```python
from build123d import *

# Parameters (mm, degrees)
SKETCH1_W           = 127
SKETCH1_H           = 61.9252
BOSS_EXTRUDE1_DEPTH = 44.45
SKETCH1_3_W         = 127
SKETCH1_3_H         = 1.8415
CUT_EXTRUDE2_DEPTH  = 38.1
SKETCH2_W           = 71.12
SKETCH2_H           = 32.258
SKETCH2_W_2         = 35.442647017
SKETCH2_H_2         = 23.182829488
CUT_EXTRUDE3_DEPTH  = 38.1
CHAMFER2_SIZE       = 10.16
CUT_EXTRUDE5_DEPTH  = 100.210800294
FILLET3_R           = 2.54
SKETCH2_3_W         = 35.442647017
SKETCH2_3_H         = 23.182829488
CUT_EXTRUDE6_DEPTH  = 84.466970107
CHAMFER3_SIZE       = 2.54


with BuildPart() as part:
    # Sketch1 → Boss-Extrude1 (new body)
    with BuildSketch(Plane(origin=(0, 0, 0), x_dir=(1, 0, 0), z_dir=(0, 1, 0))):
        Rectangle(SKETCH1_W, SKETCH1_H)
    extrude(amount=BOSS_EXTRUDE1_DEPTH)

    # Sketch1<3> → Cut-Extrude2 (cut)
    with BuildSketch(Plane(origin=(0, 0, 0), x_dir=(1, 0, 0), z_dir=(0, 1, 0))):
        with Locations((0, 23.69185)):
            Rectangle(SKETCH1_3_W, SKETCH1_3_H)
        with Locations((0, -23.69185)):
            Rectangle(SKETCH1_3_W, SKETCH1_3_H)
    extrude(amount=CUT_EXTRUDE2_DEPTH, mode=Mode.SUBTRACT)

    # Sketch2 → Cut-Extrude3 (cut)
    with BuildSketch(Plane(origin=(0, 44.45, 0), x_dir=(1, 0, 0), z_dir=(0, 1, 0))):
        with Locations((1.016, 0)):
            Rectangle(SKETCH2_W, SKETCH2_H)
        with Locations((12.504676492, 0)):
            Rectangle(SKETCH2_W_2, SKETCH2_H_2, mode=Mode.SUBTRACT)
    extrude(amount=-CUT_EXTRUDE3_DEPTH, mode=Mode.SUBTRACT)

    # Chamfer2
    chamfer2_edges = [part.edges().sort_by_distance(p)[0] for p in [
        (36.576, 44.45, 0),
        (1.016, 44.45, -16.129),
        (-34.544, 44.45, 0),
        (1.016, 44.45, 16.129),
    ]]
    chamfer(chamfer2_edges, length=CHAMFER2_SIZE)

    # Sketch7 → Cut-Extrude5 (cut, through all)
    with BuildSketch(Plane.XY.offset(30.9626)):
        Polygon((-50.795476794, 0), (-63.5, 44.45), (-63.5, 0), align=None)
        Polygon((63.5, 44.45), (50.795476794, 0), (63.5, 0), align=None)
    extrude(amount=-CUT_EXTRUDE5_DEPTH, mode=Mode.SUBTRACT)

    # Fillet3
    fillet3_edges = [part.edges().sort_by_distance(p)[0] for p in [
        (-57.147738397, 22.225, -30.9626),
        (-57.147738397, 22.225, 30.9626),
        (57.147738397, 22.225, 30.9626),
        (57.147738397, 22.225, -30.9626),
    ]]
    fillet(fillet3_edges, radius=FILLET3_R)

    # Sketch2<3> → Cut-Extrude6 (cut, through all)
    with BuildSketch(Plane(origin=(0, 44.45, 0), x_dir=(1, 0, 0), z_dir=(0, 1, 0))):
        with Locations((12.504676492, 0)):
            Rectangle(SKETCH2_3_W, SKETCH2_3_H)
    extrude(amount=-CUT_EXTRUDE6_DEPTH, mode=Mode.SUBTRACT)

    # Chamfer3
    chamfer3_edges = [part.edges().sort_by_distance(p)[0] for p in [
        (30.226, 0, 0),
        (12.504676491, 0, 11.591414744),
        (-5.216647017, 0, 0),
        (12.504676491, 0, -11.591414744),
    ]]
    chamfer(chamfer3_edges, length=CHAMFER3_SIZE)


solid = part.part
```
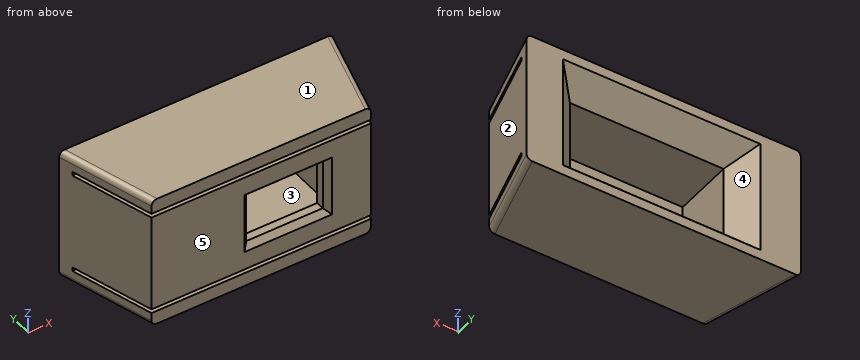
Build history of the part. All positions in model axes, mm. Face numbers are marked on the shaded views. A direction names the side the tool comes from. Round coordinates to 2 decimals unless told otherwise and drop trailing zeros. Write each loop counter-clockwise with the first axis right and the second up, starting at its lowest first coordinate (ties: lowest second). Pieces come first, ordered by that corner, then holes.
1) Band-saw the part on C-C, the plane y = 17. Give the number of separate pieces and of enclosed holes in the cut face, and give its area (3 significant figures).
2) Band-saw the part on A-A, the plane x = 23.5. List the corners of the cut face in (y, z).
3) Band-saw the part on D-D, the plane z = 20. List the corners of the cut face in (x, y) (3 decimals), and give its area (3 significant figures).
4) 3-axis set-ups, long thin cutter, end or side, ignore diameter. For the marked faces 4 and 5: which of +Z, -Z, +X, -X, +Y, -Y reach the whole face in a straight line?
5) Pin check, flat tips, straight feed: pin 1 (14 mm diameter, centred on y = 22, z = -1, fed in from -X); pin 2 (0.6 mm diameter, centred on x = 18.5, z = -23.5, fed in from -Y); pin 3 (3 mm diameter, centred on y = 4.5, z = -1, fed in from -X). Stop position of each tip, or through.
6) Band-saw the part on B-B, the plane x = -46. List the corners of the cut face in (y, z).
7) Drill centre lines: probe 1 along Z at (x, y) = (57, 37.5); probe 2 along Z at (x, y) = (-18, 15); probe 3 along Z at (x, y) = (-2, 6). Where is each one in solid material? Low to high.
8) Mould opens along X. For the marked faces 1, 2 and 3 say: +X half, -X half, draft (parallel to the pull), parting line (faces both ways), or undercut.
Ans:
1. separate pieces: 3
1. enclosed holes: 1
1. area: 4,180 mm2
2. outline: (0, -30.96) - (44.45, -30.96) - (44.45, -26.29) - (34.29, -16.13) - (6.35, -16.13) - (6.35, -11.59) - (2.54, -11.59) - (0, -14.13) - (0, -22.77) - (38.1, -22.77) - (38.1, -24.61) - (0, -24.61) - close; (0, 14.13) - (2.54, 11.59) - (6.35, 11.59) - (6.35, 16.13) - (34.29, 16.13) - (44.45, 26.29) - (44.45, 30.96) - (0, 30.96) - (0, 24.61) - (38.1, 24.61) - (38.1, 22.77) - (0, 22.77) - close
3. outline: (-63.5, 44.45) - (-50.795, 0) - (50.795, 0) - (63.5, 44.45) - (46.736, 44.45) - (40.447, 38.161) - (-38.415, 38.161) - (-44.704, 44.45) - close
3. area: 4,540 mm2
4. face 4: +Y
4. face 5: +Z, -Z, +X, -X, -Y
5. pin 1: stops at x = -59.08
5. pin 2: stops at y = 38.1
5. pin 3: stops at x = -52.51
6. outline: (0, -30.96) - (44.45, -30.96) - (44.45, 30.96) - (0, 30.96) - (0, 24.61) - (38.1, 24.61) - (38.1, 22.77) - (0, 22.77) - (0, -22.77) - (38.1, -22.77) - (38.1, -24.61) - (0, -24.61) - close
7. probe 1: z = -30.96 to -24.61, -22.77 to 22.77, 24.61 to 30.96
7. probe 2: z = -30.96 to -24.61, -22.77 to -16.13, 16.13 to 22.77, 24.61 to 30.96
7. probe 3: z = -30.96 to -24.61, -22.77 to -11.59, 11.59 to 22.77, 24.61 to 30.96
8. face 1: draft
8. face 2: +X half
8. face 3: undercut
